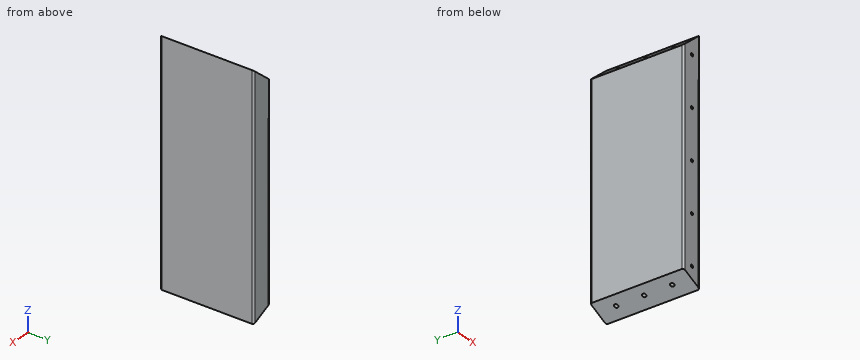
from build123d import *

# Parameters (mm, degrees)
SKETCH1_W                        = 45
SKETCH1_H                        = 200
BOSS_EXTRUDE1_DEPTH              = 510
FILLET1_R                        = 4
CUT_EXTRUDE1_DEPTH               = 549.700926986
CUT_EXTRUDE1_DEPTH_BACK          = 549.700926986
CUT_EXTRUDE2_DEPTH               = 539.19055733
CUT_EXTRUDE2_DEPTH_BACK          = 539.19055733
F_8_0MM_DOWEL_SLOT1_D            = 8
F_8_0MM_DOWEL_SLOT1_DEPTH        = 22.596557524
F_8_0MM_DOWEL_SLOT1_CSINK_D      = 8.05
F_8_0MM_DOWEL_SLOT1_CSINK_ANGLE  = 90
F_8_0MM_DOWEL_SLOT1_TIP          = 2.403442476
F_6_0MM_DOWEL_SLOT_D             = 6
F_6_0MM_DOWEL_SLOT_DEPTH         = 128.197418143
F_6_0MM_DOWEL_SLOT_CSINK_D       = 6.05
F_6_0MM_DOWEL_SLOT_CSINK_ANGLE   = 90
F_6_0MM_DOWEL_SLOT_TIP           = 1.802581857
F_6_0MM_DOWEL_SLOT4_D            = 6
F_6_0MM_DOWEL_SLOT4_DEPTH        = 10.197418143
F_6_0MM_DOWEL_SLOT4_TIP          = 1.802581857
F_6_0MM_DOWEL_SLOT17_D           = 6
F_6_0MM_DOWEL_SLOT17_DEPTH       = 28.197418143
F_6_0MM_DOWEL_SLOT17_CSINK_D     = 6.05
F_6_0MM_DOWEL_SLOT17_CSINK_ANGLE = 90
F_6_0MM_DOWEL_SLOT17_TIP         = 1.802581857


with BuildPart() as part:
    # Sketch1 → Boss-Extrude1 (new body)
    with BuildSketch(Plane.XY):
        with Locations((-8.688255411, 34.272684877)):
            Rectangle(SKETCH1_W, SKETCH1_H)
    extrude(amount=BOSS_EXTRUDE1_DEPTH)

    # Fillet1
    fillet1_edges = [part.edges().sort_by_distance(p)[0] for p in [
        (13.811744589, 134.272684877, 255),
        (13.811744589, -65.727315123, 255),
        (-31.188255411, -65.727315123, 255),
        (-31.188255411, 134.272684877, 255),
    ]]
    fillet(fillet1_edges, radius=FILLET1_R)

    # Sketch2 → Cut-Extrude1 (cut, two sides: drawn at the far end of the back side and taken through both)
    with BuildSketch(Plane(origin=(0, 134.272684877, 0), x_dir=(1, 0, 0), z_dir=(0, 1, 0)).offset(-CUT_EXTRUDE1_DEPTH_BACK)):
        Polygon((788.614470133, -1148.76248804), (13.811744589, -498.67461207), (-31.188255411, -460.917963243), (-805.990980955, 189.169912727), (-2106.166732895, -1360.435538361), (-511.561281807, -2698.367939128), align=None)
    extrude(amount=CUT_EXTRUDE1_DEPTH + CUT_EXTRUDE1_DEPTH_BACK, mode=Mode.SUBTRACT)

    # Sketch3 → Cut-Extrude2 (cut, two sides: drawn at the far end of the back side and taken through both)
    with BuildSketch(Plane(origin=(0, 134.272684877, 0), x_dir=(1, 0, 0), z_dir=(0, 1, 0)).offset(-CUT_EXTRUDE2_DEPTH_BACK)):
        Polygon((-948.658060529, -446.533100004), (-31.188255411, -20.877527163), (13.811744589, 0), (931.281549707, 425.655572841), (79.970404025, 2260.595183077), (-1799.969206211, 1388.406510232), align=None)
    extrude(amount=CUT_EXTRUDE2_DEPTH + CUT_EXTRUDE2_DEPTH_BACK, mode=Mode.SUBTRACT)

    # Ø8.0mm Dowel Slot1
    with Locations(Plane(origin=(-1225.746798414, -65.727315123, 575.087047823), x_dir=(-0.9071269657115731, 0, 0.4208570637151221), z_dir=(-0.4208570637151221, 0, -0.9071269657115731))):
        with Locations((-1339.359258027, 40), (-1339.359258027, 100), (-1339.359258027, 160)):
            CounterSinkHole(F_8_0MM_DOWEL_SLOT1_D / 2, F_8_0MM_DOWEL_SLOT1_CSINK_D / 2, depth=F_8_0MM_DOWEL_SLOT1_DEPTH, counter_sink_angle=F_8_0MM_DOWEL_SLOT1_CSINK_ANGLE)
            with Locations((0, 0, -(F_8_0MM_DOWEL_SLOT1_DEPTH + F_8_0MM_DOWEL_SLOT1_TIP / 2))):  # 118° drill point
                Cone(0, F_8_0MM_DOWEL_SLOT1_D / 2, F_8_0MM_DOWEL_SLOT1_TIP, mode=Mode.SUBTRACT)

    # Ø6.0mm Dowel Slot
    with Locations(Plane(origin=(-1255.768167205, -65.727315123, 566.463420302), x_dir=(1, 0, 0), z_dir=(0, 0, 1))):
        with Locations((1247.849951753, 160), (1247.849951753, 100), (1247.849951753, 40)):
            CounterSinkHole(F_6_0MM_DOWEL_SLOT_D / 2, F_6_0MM_DOWEL_SLOT_CSINK_D / 2, depth=F_6_0MM_DOWEL_SLOT_DEPTH, counter_sink_angle=F_6_0MM_DOWEL_SLOT_CSINK_ANGLE)
            with Locations((0, 0, -(F_6_0MM_DOWEL_SLOT_DEPTH + F_6_0MM_DOWEL_SLOT_TIP / 2))):  # 118° drill point
                Cone(0, F_6_0MM_DOWEL_SLOT_D / 2, F_6_0MM_DOWEL_SLOT_TIP, mode=Mode.SUBTRACT)

    # Ø6.0mm Dowel Slot4
    with Locations(Plane(origin=(-1324.714305528, -77.727315123, 452.529822169), x_dir=(0.642759292005894, 0, -0.766068203582476), z_dir=(0, -1, 0))):
        with Locations((-341.005231297, 740.318686522), (-261.339405676, 807.171930483), (-181.750714685, 873.960445306), (-102.007754434, 940.878418405), (-22.496198074, 1007.60220409), (847.496198074, 1007.60220409), (927.007754434, 940.878418405), (1006.750714685, 873.960445306), (1086.339405676, 807.171930483), (1166.005231297, 740.318686522)):
            Hole(F_6_0MM_DOWEL_SLOT4_D / 2, depth=F_6_0MM_DOWEL_SLOT4_DEPTH)
            with Locations((0, 0, -(F_6_0MM_DOWEL_SLOT4_DEPTH + F_6_0MM_DOWEL_SLOT4_TIP / 2))):  # 118° drill point
                Cone(0, F_6_0MM_DOWEL_SLOT4_D / 2, F_6_0MM_DOWEL_SLOT4_TIP, mode=Mode.SUBTRACT)

    # Ø6.0mm Dowel Slot17
    with Locations(Plane(origin=(-1324.714305529, -77.727315123, 452.529822169), x_dir=(0.642759292005894, 0, -0.766068203582476), z_dir=(0, -1, 0))):
        with Locations((22.5, 1726.5), (22.5, 1640.5), (802.5, 1726.5), (802.5, 1640.5), (22.5, -955.960621131), (22.5, -1636.5), (802.5, -1462.5), (802.5, -1636.5), (22.5, -1722.5), (802.5, -1722.5), (22.5, -1550.5), (802.5, -640.31), (120, -1722.5), (217.5, -1722.5), (315, -1722.5), (412.5, -1722.5), (510, -1722.5), (607.5, -1722.5), (705, -1722.5), (22.5, -861.25), (22.5, -883.75), (-22.496198074, -917.60220409), (802.5, -861.25), (802.5, -883.75), (847.496198074, -917.60220409), (802.5, -529.84), (22.5, -750.249617159), (-341.005231297, -650.318686522), (1166.005231297, -650.318686522), (-310.084924074, 22.5), (-310.084924074, 67.5), (22.5, 67.5), (22.5, 22.5), (802.5, 67.5), (802.5, 22.5), (1133.730020848, 67.5), (1133.730020848, 22.5), (1166.005231297, 740.318686522), (802.560751791, 973.75), (802.560751791, 951.25), (847.496198074, 1007.60220409), (-22.496198074, 1007.60220409), (22.560751791, 951.25), (-341.005231297, 740.318686522), (22.5, 1812.5), (802.5, 1812.5), (22.5, 1552.5), (802.5, 1552.5), (-102.162023695, -850.748960129), (-181.827849315, -783.895716167), (-261.493674936, -717.042472206), (927.162023695, -850.748960129), (1006.827849315, -783.895716167), (1086.493674936, -717.042472206), (1086.493674936, 807.042472206), (1006.827849315, 873.895716167), (927.162023695, 940.748960129), (-102.162023695, 940.748960129), (-181.827849315, 873.895716167), (-261.493674936, 807.042472206), (-199.224924074, 67.5), (-88.364924074, 67.5), (-199.224924074, 22.5), (-88.364924074, 22.5), (912.010020848, 67.5), (1022.870020848, 67.5), (912.010020848, 22.5), (1022.870020848, 22.5), (120, 67.5), (217.5, 67.5), (315, 67.5), (607.5, 67.5), (705, 67.5), (510, 67.5), (120, 22.5), (217.5, 22.5), (315, 22.5), (510, 22.5), (607.5, 22.5), (705, 22.5), (412.5, 22.5), (22.5, -750.78), (22.5, -640.31), (22.5, -529.84), (22.5, -419.37), (22.5, -308.9), (22.5, -198.43), (22.5, -87.96), (802.5, -750.78), (802.5, -419.37), (802.5, -308.9), (802.5, -198.43), (22.5, 177.97), (22.5, 288.44), (22.5, 398.91), (22.5, 509.38), (22.5, 619.85), (22.5, 730.32), (22.5, 840.79), (802.5, -87.96), (802.5, 177.97), (802.5, 288.44), (120.000330201, 1812.753749877), (217.5, 1812.5), (315, 1812.5), (412.5, 1812.5), (510, 1812.5), (607.5, 1812.5), (705, 1812.5), (120.060751791, 951.25), (217.560751791, 951.25), (315.060751791, 951.25), (412.560751791, 951.25), (510.060751791, 951.25), (607.560751791, 951.25), (705.060751791, 951.25), (656.310751791, 973.75), (558.810751791, 973.75), (461.310751791, 973.75), (363.810751791, 973.75), (266.310751791, 973.75), (168.810751791, 973.75), (120, -861.25), (217.5, -861.25), (315, -861.25), (412.5, -861.25), (510, -861.25), (607.5, -861.25), (705, -861.25), (656.25, -883.75), (558.75, -883.75), (461.25, -883.75), (168.75, -883.75), (266.25, -883.75), (363.75, -883.75), (802.560751791, -955.960621131), (412.5, 67.5), (802.5, 730.32), (802.560751791, 840.79), (802.5, 398.91), (802.5, 509.38), (802.5, 619.85), (-360.000025903, 699.425529794), (-360.000025903, -609.521258848), (-360.000025903, 598.725529794), (-360.000025903, 498.025529794), (-360.000025903, 397.325529794), (-360.000025903, 296.625529794), (-360.000025903, 195.925529794), (-360.000025903, 95.225529794), (-360.000025903, -5.474470206), (-360.000025903, -106.174470206), (-360.000025903, -206.874470206), (-360.000025903, -307.574470206), (-360.000025903, -408.274470206), (-360.000025903, -508.974470206), (1185.00101945, 699.425529452), (1185.000941829, 598.725529794), (1185.000864209, 498.025529794), (1185.000708968, 296.625529794), (1185.000631348, 195.925529794), (1185.000553727, 95.225529794), (1185.000476107, -5.474470206), (1185.000398486, -106.174470206), (1185.000320866, -206.874470206), (1185.000165625, -408.274470206), (1185.000088004, -508.974470206), (1185.000786589, 397.325529794), (22.560751791, 1016.385842825), (802.560751791, 1016.385842825), (802.560751791, -1550.5), (22.560751791, 973.75), (802.560751791, -363.966698641)):
            CounterSinkHole(F_6_0MM_DOWEL_SLOT17_D / 2, F_6_0MM_DOWEL_SLOT17_CSINK_D / 2, depth=F_6_0MM_DOWEL_SLOT17_DEPTH, counter_sink_angle=F_6_0MM_DOWEL_SLOT17_CSINK_ANGLE)
            with Locations((0, 0, -(F_6_0MM_DOWEL_SLOT17_DEPTH + F_6_0MM_DOWEL_SLOT17_TIP / 2))):  # 118° drill point
                Cone(0, F_6_0MM_DOWEL_SLOT17_D / 2, F_6_0MM_DOWEL_SLOT17_TIP, mode=Mode.SUBTRACT)


solid = part.part
Geometry check sheet. Reference: the model listing, model coordinates, mm. Give positions to 0.01 mm unless a question says otherwise; leave off trailing zeros. Loops run counter-clockwise (first coordinate to the right, second up) from the corner with the lowest first, then second, coordinate; pieces in that order, holes last. Notation, with made-up numbers: M -29,31.5 L -15,31.5 A21 cw -15,43.5 Z; hole C 34,70 d11. An arc over 180 degrees is marked long. Write each question's results on one line, items separated by ' | '.
1) Section check A-A, the plane y = 74. Record the boundary of the cut face in (x, z), plus the area to 3 significant figures.
Answers follow:
outline: M -31.19,20.88 L 13.81,0 L 13.81,498.67 L -31.19,460.92 Z | area: 21,100 mm2
2) Gauge pin test, flat ends, axial feed: pin 1 (12 mm diameter, centred on x = -5, y = -30.5, fed in from +Z); pin 2 (3.5 mm diameter, centred on x = -7.92, y = 94.27, fed in from -Z); pin 3 (2 mm diameter, centred on x = 6, y = 24.5, fed in from +Z). Record the tip position at first contact, or that the pin passes through.
Answers follow:
pin 1: z = 487.93 | pin 2: z = 9.27 | pin 3: z = 492.96
3) Thickness scan on line 1 (Y direction, x = 10.5, z = 217.5); line 2 (Z direction, x = -29, y = 45); line 3 (Z direction, x = 1, y = 18). Record the ranges inside material, lowest first.
Answers follow:
line 1: -65.67 to 134.21 | line 2: 19.86 to 462.75 | line 3: 5.94 to 487.93
